Part model, mm, in its own coordinate system. Face numbers are marked on the shaded views. A direction names the side the tool comes from. Round coordinates to 2 decimals unless told otherwise and drop trailing zeros. Loops run counter-clockwise (first coordinate to the right, second up) from the corner with the lowest first, then second, coordinate; pieces in that order, holes last.
(1) Probe probe 1 along Z at (x, y) = (-9, -31); probe 2 along Y at (x, z) = (2.5, 17.5); probe 3 along Y at (x, z) = (-5, 25). List the from-to ranges inside material, lowest first.
(2) Tool access for the marked faces 1 and 2: list every direction of +Z, -Z, +X, -X, +Y, -Y with a clear straight run to the whole face (end or side of a thin tool).
(3) Cut at B-B on y = 3.5. List the corners of the cut face in (x, z).
(4) Cut at A-A on x = 0. List the corners of the cut face in (y, z), then the cut area to 3 significant figures.
(5) Cut at C-C on z = 39.5. List the corners of the cut face in (x, y).
(6) Flat gauge pins, fed straight in: pin 1 (8 mm diameter, centred on y = -24.5, z = 36, fed in from +X); pin 2 (8 mm diameter, centred on x = -8, z = 12, fed in from +Y); pin 3 (4 mm diameter, centred on y = 24, z = 38.5, fed in from +X); pin 4 (3.5 mm diameter, centred on x = -0.5, y = -36.5, fed in from -Z). Where does each tip first touch, or does it go through?
(7) Cut at D-D on x = 24. List the corners of the cut face in (y, z), then the cut area to 3 significant figures.
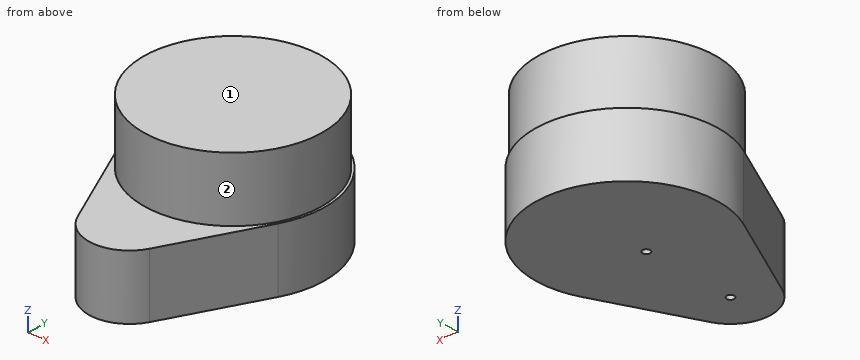
from build123d import *

# Parameters (mm, degrees)
EXTRUDE_1_DEPTH           = 25
SKETCH_2_R                = 35
EXTRUDE_2_DEPTH           = 25
HOLE_WIZARD_3_0_3_1_D     = 3
HOLE_WIZARD_3_0_3_1_DEPTH = 5


with BuildPart() as part:
    # 草图1 → 凸台-拉伸1 (new body)
    with BuildSketch(Plane.XY.offset(20)):
        with BuildLine():
            Line((14.371408237, -44.032967033), (32.335668533, -7.324175824))
            ThreePointArc((32.335668533, -7.324175824), (0, 44.5), (-32.335668533, -7.324175824))
            Line((-32.335668533, -7.324175824), (-14.371408237, -44.032967033))
            ThreePointArc((-14.371408237, -44.032967033), (0, -53), (14.371408237, -44.032967033))
        make_face()
    extrude(amount=-EXTRUDE_1_DEPTH)

    # 草图2 → 凸台-拉伸2 (add)
    with BuildSketch(Plane(origin=(0, 0, 20), x_dir=(-1, 0, 0), z_dir=(0, 0, -1))):
        with Locations(Location((0, 8.5, 0), (0, 0, 180))):
            Circle(SKETCH_2_R)
    extrude(amount=-EXTRUDE_2_DEPTH)

    # Ø3.0 (3) 直径孔1
    with Locations(Plane(origin=(0, 0, -5), x_dir=(-1, 0, 0), z_dir=(0, 0, -1))):
        with Locations((0, 0), (0, -37)):
            Hole(HOLE_WIZARD_3_0_3_1_D / 2, depth=HOLE_WIZARD_3_0_3_1_DEPTH)


solid = part.part
Final values:
1. probe 1: z = -5 to 20
1. probe 2: y = -52.8 to 44.41
1. probe 3: y = -26.14 to 43.14
2. face 1: +Z, +X, -X, +Y, -Y
2. face 2: +Z
3. outline: (-35.65, -5) - (35.65, -5) - (35.65, 20) - (34.64, 20) - (34.64, 45) - (-34.64, 45) - (-34.64, 20) - (-35.65, 20) - close
4. outline: (-53, -5) - (-38.5, -5) - (-38.5, 0) - (-35.5, 0) - (-35.5, -5) - (-1.5, -5) - (-1.5, 0) - (1.5, 0) - (1.5, -5) - (44.5, -5) - (44.5, 20) - (43.5, 20) - (43.5, 45) - (-26.5, 45) - (-26.5, 20) - (-53, 20) - close
4. area: 4,160 mm2
5. outline: circle Ø70 at (0, 8.5)
6. pin 1: stops at x = 19.6
6. pin 2: stops at y = 44.28
6. pin 3: stops at x = 32.29
6. pin 4: stops at z = -5
7. outline: (-24.36, -5) - (35.33, -5) - (35.33, 20) - (33.98, 20) - (33.98, 45) - (-16.98, 45) - (-16.98, 20) - (-24.36, 20) - close
7. area: 2,770 mm2
